Check sheet for the modelled part. Datum: model origin and axes. Units: mm. A direction names the side the tool comes from. Coordinates: 2 decimals unless noted, no trailing zeros. Order: outer loops, then holes, each group sorted by start corner. A loop starts at its lowest first (then second) coordinate and runs counter-clockwise, first axis right, second up.
1. Thickness scan on line 1 (X direction, y = 6.8, z = 1.05); line 2 (Y direction, x = -83, z = 1.2); line 3 (X direction, y = 28.5, z = 0.25). Record the ranges inside material, lowest first.
2. Gauge pin test, flat end, axial feed: pin 1 Ø1.7 at (x, y) = (-67.87, 23.2) entering from -Z. Record the tip position at first contact, or that the pin passes through.
3. Draft check along Y on faces 3 (the flat face through (-1, 35, 1)), 4 (the flat face through (-1, -35, 1)), 5 (the flat face through (-1, 0, 3)), 6 (the cylindrical face through (84.1, 0.45, 1.48)). Enter one of: released by +Y, released by -Y, zero draft, split by the parting line, or undercut.
4. Cross-section at A-A (x = 60.17). Enter the section's corners in (y, z).
5. Set-up check for faces 1 (the flat face through (-85.17, 22, 1)), 2 (the flat face through (90.17, 0, 1)): record each of +Z, -Z, +X, -X, +Y, -Y from which the full face is reachable in a straight line by a thin tool's end or side.
6. Cross-section at C-C (x = 31). Enter the section's corners in (y, z).
7. Cross-section at B-B (z = 0.65). Count the separate pieces of the cut face and the enclosed holes in it, then the cut area to 3 significant figures.
```python
from build123d import *

# Parameters (mm, degrees)
SCHIZZO1_W                   = 180.34
SCHIZZO1_H                   = 70
ESTRUSIONE_ESTRUSIONE1_DEPTH = 3
SCHIZZO2_R                   = 1.5
SCHIZZO2_W                   = 5
SCHIZZO2_H                   = 15
TAGLIO_ESTRUSIONE1_DEPTH     = 4
SCHIZZO3_R                   = 7.94
SCHIZZO3_R_2                 = 1.05
TAGLIO_ESTRUSIONE2_DEPTH     = 4


with BuildPart() as part:
    # Schizzo1 → Estrusione-Estrusione1 (new body)
    with BuildSketch(Plane.XY):
        Rectangle(SCHIZZO1_W, SCHIZZO1_H)
    extrude(amount=ESTRUSIONE_ESTRUSIONE1_DEPTH)

    # Schizzo2 → Taglio-Estrusione1 (cut, through all)
    with BuildSketch(Plane.XY):
        with Locations((-82.67, 0)):
            Circle(SCHIZZO2_R)
        with Locations((82.67, 0)):
            Circle(SCHIZZO2_R)
        with Locations((-82.67, 22.5)):
            Rectangle(SCHIZZO2_W, SCHIZZO2_H)
        with Locations((-82.67, -22.5)):
            Rectangle(SCHIZZO2_W, SCHIZZO2_H)
        with Locations((82.67, 22.5)):
            Rectangle(SCHIZZO2_W, SCHIZZO2_H)
        with Locations((82.67, -22.5)):
            Rectangle(SCHIZZO2_W, SCHIZZO2_H)
    extrude(amount=TAGLIO_ESTRUSIONE1_DEPTH, mode=Mode.SUBTRACT)

    # Schizzo3 → Taglio-Estrusione2 (cut, through all)
    with BuildSketch(Plane.XY):
        with Locations((-60.17, 15)):
            Circle(SCHIZZO3_R)
        with Locations((-34.67, 15)):
            Circle(SCHIZZO3_R)
        with Locations((60.17, 15)):
            Circle(SCHIZZO3_R)
        with Locations((34.67, 15)):
            Circle(SCHIZZO3_R)
        with Locations((-26.97, 6.8)):
            Circle(SCHIZZO3_R_2)
        with Locations((-26.97, 23.2)):
            Circle(SCHIZZO3_R_2)
        with Locations((-67.87, 6.8)):
            Circle(SCHIZZO3_R_2)
        with Locations((-67.87, 23.2)):
            Circle(SCHIZZO3_R_2)
        with Locations((26.97, 23.2)):
            Circle(SCHIZZO3_R_2)
        with Locations((26.97, 6.8)):
            Circle(SCHIZZO3_R_2)
        with Locations((67.87, 6.8)):
            Circle(SCHIZZO3_R_2)
        with Locations((67.87, 23.2)):
            Circle(SCHIZZO3_R_2)
    extrude(amount=TAGLIO_ESTRUSIONE2_DEPTH, mode=Mode.SUBTRACT)


solid = part.part
```
Data:
1. line 1: x = -90.17 to -68.92, -66.82 to -28.02, -25.92 to 25.92, 28.02 to 66.82, 68.92 to 90.17
1. line 2: y = -35 to -30, -15 to -1.46, 1.46 to 15, 30 to 35
1. line 3: x = -90.17 to -85.17, -80.17 to 80.17, 85.17 to 90.17
2. pin 1: passes through
3. face 3: released by +Y
3. face 4: released by -Y
3. face 5: zero draft
3. face 6: undercut
4. outline: (-35, 0) - (7.06, 0) - (7.06, 3) - (-35, 3) - close; (22.94, 0) - (35, 0) - (35, 3) - (22.94, 3) - close
5. face 1: +Z, -Z
5. face 2: +Z, -Z, +X, +Y, -Y
6. outline: (-35, 0) - (7.96, 0) - (7.96, 3) - (-35, 3) - close; (22.04, 0) - (35, 0) - (35, 3) - (22.04, 3) - close
7. separate pieces: 1
7. enclosed holes: 18
7. area: 11,500 mm2
